For this review, take the finished solid that the model builds, in its own axes (mm). A direction names the side the tool comes from. Give positions to 0.01 mm unless a question says otherwise; leave off trailing zeros. Loops run counter-clockwise (first coordinate to the right, second up) from the corner with the lowest first, then second, coordinate; pieces in that order, holes last. Notation, with made-up numbers: (45.25, -38.5) -> (68.25, -38.5) arc R26 cw to (68.25, -10.5) -> close; hole circle Ø7 at (20.5, 80). An arc over 180 degrees is marked (long way). Write each question's results on one line, items separated by ' | '. Start each with the question number.
```python
from build123d import *

# Parameters (mm, degrees)
SKETCH1_R             = 17.5
BOSS_EXTRUDE1_DEPTH   = 5
F_3_0MM_DOWEL_HOLE1_D = 3
M3X0_5_TAPPED_HOLE1_D = 2.5
SKETCH10_R            = 12.5
BOSS_EXTRUDE2_DEPTH   = 23
CHAMFER1_SIZE         = 0.3
KEYWAY_DEPTH          = 39.539297239
FILLET1_R             = 1


with BuildPart() as part:
    # Sketch1 → Boss-Extrude1 (new body)
    with BuildSketch(Plane.XY):
        with Locations((100, 0)):
            Circle(SKETCH1_R)
    extrude(amount=BOSS_EXTRUDE1_DEPTH)

    # Ø3.0mm Dowel Hole1 (through all)
    with Locations(Plane(origin=(0, 0, 0), x_dir=(-1, 0, 0), z_dir=(0, 0, -1))):
        with Locations((-100, 15)):
            Hole(F_3_0MM_DOWEL_HOLE1_D / 2)

    # M3x0.5 Tapped Hole1 (through all)
    with Locations(Plane(origin=(0, 0, 0), x_dir=(-1, 0, 0), z_dir=(0, 0, -1))):
        with Locations((-110.606601718, 10.606601718), (-89.393398282, 10.606601718), (-110.606601718, -10.606601718), (-89.393398282, -10.606601718)):
            Hole(M3X0_5_TAPPED_HOLE1_D / 2)

    # Sketch10 → Boss-Extrude2 (add)
    with BuildSketch(Plane.XY.offset(5)):
        with Locations((100, 0)):
            Circle(SKETCH10_R)
    extrude(amount=BOSS_EXTRUDE2_DEPTH)

    # Chamfer1
    chamfer1_edges = [part.edges().sort_by_distance(p)[0] for p in [
        (88.143398282, -10.606601718, 0),
        (82.5, 0, 0),
        (109.356601718, -10.606601718, 0),
        (88.143398282, 10.606601718, 0),
        (109.356601718, 10.606601718, 0),
        (87.5, 0, 28),
        (82.5, 0, 5),
        (98.5, 15, 0),
    ]]
    chamfer(chamfer1_edges, length=CHAMFER1_SIZE)

    # KeySketch → Keyway (cut, through all)
    with BuildSketch(Plane(origin=(101.36896109, 1.08062806, 28), x_dir=(1, 0, 0), z_dir=(0, 0, 1))):
        with BuildLine():
            Line((-3.86896109, 6.518714017), (-3.86896109, 9.21937194))
            Line((-3.86896109, 9.21937194), (1.13103891, 9.21937194))
            Line((1.13103891, 9.21937194), (1.13103891, 6.518714017))
            ThreePointArc((1.13103891, 6.518714017), (-1.36896109, -9.08062806), (-3.86896109, 6.518714017))
        make_face()
    extrude(amount=-KEYWAY_DEPTH, mode=Mode.SUBTRACT)

    # Fillet1
    fillet1_edges = [part.edges().sort_by_distance(p)[0] for p in [
        (87.5, 0, 5),
    ]]
    fillet(fillet1_edges, radius=FILLET1_R - 0.0001)  # a hair under: the kernel refuses the full size


solid = part.part
```
1. Draft analysis for pull direction X (two halves, no side actions). For faces 4 (the cylindrical face through (111.8, 10.98, 2.68)), 5 (the cylindrical face through (111.923, 3.755, 16.698)), 6 (the flat face through (103.6, -7.4, 0)), state which applies: released by +X, released by -X, zero draft, split by the parting line, or undercut.
2. Machinability: for faces 1 (the flat face through (97.5, 9, 14)), 2 (the flat face through (105, -13, 5)), 3 (the flat face through (103, -8, 28)), which of the approach directions +Z, -Z, +X, -X, +Y, -Y give a long, thin tool a straight path to every point of the face, cutting with its end or side? Answer none if there is none.
3. For pin 1 Ø3 at (x, y) = (89.39, 10.61) entering from +Z; pin 2 Ø1.5 at (x, z) = (97.5, 11.5) entering from +Y; pin 3 Ø2.5 at (x, z) = (101, 15) entering from -Y, all flat-tipped, find the tip position at first contact; note any pin that passes through.
4. We need section B-B (z = 14). Write out the cut boundary in (x, y).
5. We need section C-C (x = 100). Count the separate pieces of the cut face and the enclosed holes in it, plus the area to 3 significant figures.
6. Wall thickness on L1, parallel to Y at x = 100, z = 1.4; L2, parallel to X at y = 1.5, z = 11; L3, parallel to Z at x = 104, y = -13: over which ranges is each line inside the solid? List them lowest first.
7. We need section A-A (y = 0). Write out the cut boundary in (x, z), plus the area to 3 significant figures.
Response:
1) face 4: undercut | face 5: split by the parting line | face 6: zero draft
2) face 1: +Z, -Z | face 2: +Z | face 3: +Z, +X, -X, +Y, -Y
3) pin 1: stops at z = 5 | pin 2: stops at y = 12.38 | pin 3: stops at y = -12.5
4) outline: circle Ø25 at (100, 0); hole (97.5, 7.6) arc R8 ccw (long way) to (102.5, 7.6) -> (102.5, 10.3) -> (97.5, 10.3) -> close
5) separate pieces: 3 | enclosed holes: 0 | area: 223 mm2
6) L1: y = -17.5 to -8, 10.3 to 13.5, 16.5 to 17.5 | L2: x = 87.59 to 92.14, 107.86 to 112.41 | L3: z = 0 to 5
7) outline: (82.5, 0.3) -> (82.8, 0) -> (92, 0) -> (92, 28) -> (87.8, 28) -> (87.5, 27.7) -> (87.5, 6) arc R1 cw to (86.5, 5) -> (82.8, 5) -> (82.5, 4.7) -> close; (108, 0) -> (117.2, 0) -> (117.5, 0.3) -> (117.5, 4.7) -> (117.2, 5) -> (113.5, 5) arc R1 cw to (112.5, 6) -> (112.5, 27.7) -> (112.2, 28) -> (108, 28) -> close | area: 302 mm2
